from build123d import *

# Parameters (mm, degrees)
SKETCH1_W           = 21.7
SKETCH1_H           = 40
BOSS_EXTRUDE1_DEPTH = 13
SKETCH3_W           = 21.7
SKETCH3_H           = 33
CUT_EXTRUDE1_DEPTH  = 9
SKETCH5_W           = 5.6
SKETCH5_H           = 9
CUT_EXTRUDE2_DEPTH  = 42.57992304
SKETCH6_R           = 2.4
CUT_EXTRUDE4_DEPTH  = 47.388468395


with BuildPart() as part:
    # Sketch1 → Boss-Extrude1 (new body)
    with BuildSketch(Plane(origin=(0, 0, 0), x_dir=(1, 0, 0), z_dir=(0, 1, 0))):
        with Locations((10.85, -20)):
            Rectangle(SKETCH1_W, SKETCH1_H)
    extrude(amount=BOSS_EXTRUDE1_DEPTH)

    # Sketch3 → Cut-Extrude1 (cut)
    with BuildSketch(Plane(origin=(0, 13, 0), x_dir=(1, 0, 0), z_dir=(0, 1, 0))):
        with Locations((10.85, -16.5)):
            Rectangle(SKETCH3_W, SKETCH3_H)
    extrude(amount=-CUT_EXTRUDE1_DEPTH, mode=Mode.SUBTRACT)

    # Sketch5 → Cut-Extrude2 (cut, through all)
    with BuildSketch(Plane(origin=(0, 0, 33), x_dir=(-1, 0, 0), z_dir=(0, 0, -1))):
        with Locations((-13.2, 8.5)):
            Rectangle(SKETCH5_W, SKETCH5_H)
    extrude(amount=-CUT_EXTRUDE2_DEPTH, mode=Mode.SUBTRACT)

    # Sketch6 → Cut-Extrude4 (cut, through all)
    with BuildSketch(Plane(origin=(0, 4, 0), x_dir=(1, 0, 0), z_dir=(0, 1, 0))):
        with Locations(Location((8.5, -12, 0), (0, 0, 270))):
            Circle(SKETCH6_R)
    extrude(amount=-CUT_EXTRUDE4_DEPTH, mode=Mode.SUBTRACT)


solid = part.part
The model under review builds one solid part; all positions refer to its coordinate system, in mm. A direction names the side the tool comes from. Coordinates: 2 decimals unless noted, no trailing zeros. Write each loop counter-clockwise with the first axis right and the second up, starting at its lowest first coordinate (ties: lowest second). Pieces come first, ordered by that corner, then holes. Notation, with made-up numbers: (-17, -18.75) - (21, -18.75) arc R15 ccw to (21, 2.25) - close; hole circle Ø6 at (71, 56.25). An arc over 180 degrees is marked (long way). Answer as a JSON object with one key per item and string values. Group by question number.
1. Add section A-A (y = 10.75). Give the boundary of the cut face in (x, z), plus the area to 3 significant figures.
2. Add section D-D (y = 3.5). Give the boundary of the cut face in (x, z), plus the area to 3 significant figures.
3. Add section B-B (x = 8.5). Give the boundary of the cut face in (y, z), plus the area to 3 significant figures.
4. Mouldability with a two-part tool opening along X and no side actions: class faces 1 (the face through (0, 3.5, 24.7)), 2 (the face through (11, 2, 0)), 3 (the face through (21.7, 3.5, 24.7)), 4 (the face through (10.88, 2.03, 11.69)) as pulls with the +X half, pulls with the -X half, needs draft (parallel to the pull), parting line crosses it, or undercut.
5. Clearance check with flat-ended pins moving along their axes: pin 1 Ø4.5 at (x, y) = (20, 10) entering from -Z; pin 2 Ø3.5 at (y, z) = (7.5, 36.5) entering from -X; pin 3 Ø3 at (x, z) = (14, 9) entering from +Y. State where each tip first meets the part, or that it passes through.
6. Machinability: for faces 5 (the face through (19, 13, 36)), 6 (the face through (5, 9, 33)), 7 (the face through (16, 8, 36)), which of the approach directions +Z, -Z, +X, -X, +Y, -Y give a long, thin tool a straight path to every point of the face, cutting with its end or side? Answer none if there is none.
7. To check wall thickness, follow probe 1 along X at (y, z) = (1.5, 12); probe 2 along Y at (x, z) = (6.25, 3.5); probe 3 along Z at (x, y) = (9.5, 7.25). State the ranges of each line that lie inside material, in increasing order.
8. Add section C-C (z = 12). Give the boundary of the cut face in (x, y).
Findings:
{
 "1": {"outline": "(0, 33) - (10.4, 33) - (10.4, 40) - (0, 40) - close; (16, 33) - (21.7, 33) - (21.7, 40) - (16, 40) - close", "area": "113 mm²"},
 "2": {"outline": "(0, 0) - (21.7, 0) - (21.7, 40) - (0, 40) - close; hole circle Ø4.8 at (8.5, 12)", "area": "850 mm²"},
 "3": {"outline": "(0, 0) - (4, 0) - (4, 9.6) - (0, 9.6) - close; (0, 14.4) - (4, 14.4) - (4, 33) - (13, 33) - (13, 40) - (0, 40) - close", "area": "204 mm²"},
 "4": {"face 1": "pulls with the -X half", "face 2": "needs draft", "face 3": "pulls with the +X half", "face 4": "undercut"},
 "5": {"pin 1": "z = 33", "pin 2": "x = 0", "pin 3": "y = 4"},
 "6": {"face 5": "+Z, -Z, +X, -X, +Y", "face 6": "-Z, +X, -X, +Y", "face 7": "+Z, -Z, +Y"},
 "7": {"probe 1": "0 to 6.1, 10.9 to 21.7", "probe 2": "0 to 4", "probe 3": "33 to 40"},
 "8": {"outline": "(0, 0) - (6.1, 0) - (6.1, 4) - (0, 4) - close; (10.9, 0) - (21.7, 0) - (21.7, 4) - (10.9, 4) - close"}
}
